```python
from build123d import *

# Parameters (mm, degrees)
SKETCH1_R                      = 6.35
BOSS_EXTRUDE1_DEPTH            = 54.102
SKETCH3_W                      = 6.35
SKETCH3_H                      = 14.605
CUT_EXTRUDE1_DEPTH             = 55.842241056
F_3_16_0_1875_DIAMETER_HOLE1_D = 4.7625
SKETCH7_RX                     = 6.35
SKETCH7_RY                     = 3.175
CUT_EXTRUDE2_DEPTH             = 56.532701566
CUT_EXTRUDE2_DEPTH_BACK        = 56.532701566
SKETCH9_W                      = 25.4
SKETCH9_H                      = 12.7


with BuildPart() as part:
    # Sketch1 → Boss-Extrude1 (new body)
    with BuildSketch(Plane(origin=(0, 0, 0), x_dir=(1, 0, 0), z_dir=(0, 1, 0))):
        with Locations(Location((0, 0, 0), (0, 0, 270))):
            Circle(SKETCH1_R)
    extrude(amount=BOSS_EXTRUDE1_DEPTH)

    # Sketch2 → Cut-Revolve1 (revolve, cut)
    with BuildSketch(Plane.XY, mode=Mode.PRIVATE) as cut_revolve1_sk:
        Polygon((26.057124612, 38.1), (6.35, 38.1), (2.54, 34.29), (2.54, 12.065), (6.35, 8.255), (26.057124612, 8.255), align=None)
    revolve(cut_revolve1_sk.sketch.rotate(Axis((0, 0, 0), (0, 1, 0)), 90), axis=Axis((0, 0, 0), (0, 1, 0)), mode=Mode.SUBTRACT)

    # Sketch3 → Cut-Extrude1 (cut, symmetric)
    with BuildSketch(Plane.XY):
        with Locations((7.62, 7.3025)):
            Rectangle(SKETCH3_W, SKETCH3_H)
    cut_extrude1 = extrude(amount=CUT_EXTRUDE1_DEPTH, both=True, mode=Mode.SUBTRACT)

    # Mirror1: Cut-Extrude1 across plane
    add(cut_extrude1.mirror(Plane(origin=(0, 0, 0), x_dir=(0, 0, 1), z_dir=(1, 0, 0))), mode=Mode.SUBTRACT)

    # 3/16 (0.1875) Diameter Hole1 (through all)
    with Locations(Plane.ZY.offset(4.445)):
        with Locations((0, 6.35)):
            Hole(F_3_16_0_1875_DIAMETER_HOLE1_D / 2)

    # Sketch7 → Cut-Revolve2 (revolve, cut)
    with BuildSketch(Plane.XY, mode=Mode.PRIVATE) as cut_revolve2_sk:
        with Locations(Location((7.9375, 46.1645), (0, 0, -90))):
            Ellipse(SKETCH7_RX, SKETCH7_RY)
    revolve(cut_revolve2_sk.sketch.rotate(Axis((0, 0, 0), (0, 1, 0)), 90), axis=Axis((0, 0, 0), (0, 1, 0)), mode=Mode.SUBTRACT)

    # Sketch8 → Cut-Revolve3 (revolve, cut)
    with BuildSketch(Plane(origin=(0, 0, 0), x_dir=(0, 0, -1), z_dir=(1, 0, 0))):
        with BuildLine():
            Line((4.7625, 54.102), (-4.7625, 54.102))
            ThreePointArc((-4.7625, 54.102), (0, 49.3395), (4.7625, 54.102))
        make_face()
    revolve(axis=Axis((0, 54.102, -4.7625), (0, 0, 1)), mode=Mode.SUBTRACT)

    # Sketch9 → Cut-Extrude2 (cut, two sides: drawn at the far end of the back side and taken through both)
    with BuildSketch(Plane(origin=(4.445, 0, 0), x_dir=(0, 0, -1), z_dir=(1, 0, 0)).offset(-CUT_EXTRUDE2_DEPTH_BACK)):
        with Locations((1.492425813, -3.81)):
            Rectangle(SKETCH9_W, SKETCH9_H)
    extrude(amount=CUT_EXTRUDE2_DEPTH + CUT_EXTRUDE2_DEPTH_BACK, mode=Mode.SUBTRACT)


solid = part.part
```
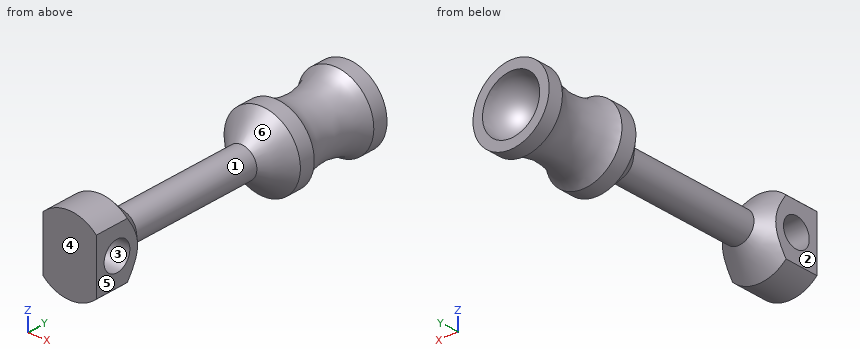
For this review, take the finished solid that the model builds, in its own axes (mm). Face numbers are marked on the shaded views. A direction names the side the tool comes from. Coordinates: 2 decimals unless noted, no trailing zeros. Write each loop counter-clockwise with the first axis right and the second up, starting at its lowest first coordinate (ties: lowest second). Pieces come first, ordered by that corner, then holes.
(1) The part is to be moulded in two halves that separate along Y. For the marked faces 4, 5 and 6, say which applies: +Y half, -Y half, draft (parallel to the pull), parting line (faces both ways), or undercut.
(2) Tool access review of the marked faces 1, 2 and 3: name each direction out of +Z, -Z, +X, -X, +Y, -Y from which nothing blocks a thin tool from reaching the whole face with its end or side.
(3) For pin 1 Ø1.5 at (x, y) = (1.5, 42) entering from +Z; pin 2 Ø3 at (x, y) = (0.5, 46.5) entering from -Z; pin 3 Ø2.5 at (y, z) = (8, -1.5) entering from -X (3 decimals); pin 4 Ø3 at (y, z) = (6.35, 0) entering from +X, all flat-tipped, find the tip position at first contact; note any pin that passes through.
(4) Add section B-B on x = 3.75. Count the separate pieces of the cut face and the enclosed holes in it, then the cut area to 3 significant figures.
(5) Add section C-C on y = 23. Give the boundary of the cut face in (x, z).
(6) Add section A-A on y = 6.35. Give the boundary of the cut face in (x, z) (3 decimals).
(7) Wall thickness on probe 1 along Y at (x, z) = (-3.75, 2) (3 decimals); probe 2 along Y at (x, z) = (-2.25, -1.5); probe 3 along Y at (x, z) = (0, 0): over which ranges is each line inside the solid? List them lowest first.
Answer sheet:
1. face 4: -Y half
1. face 5: draft
1. face 6: undercut
2. face 1: none
2. face 2: +Z, -Z, -X, -Y
2. face 3: +X, -X
3. pin 1: stops at z = 5.77
3. pin 2: stops at z = -4.89
3. pin 3: stops at x = -4.445
3. pin 4: passes through
4. separate pieces: 2
4. enclosed holes: 1
4. area: 192 mm2
5. outline: circle Ø5.08 at (0, 0)
6. outline: (-4.445, -4.535) arc R6.35 ccw to (4.445, -4.535) - (4.445, -2.381) - (-4.445, -2.381) - close; (-4.445, 2.381) - (4.445, 2.381) - (4.445, 4.535) arc R6.35 ccw to (-4.445, 4.535) - close
7. probe 1: y = 2.54 to 5.058, 7.642 to 10.355, 36 to 51.953
7. probe 2: y = 2.54 to 4.5, 8.2 to 11.9, 34.45 to 50.18
7. probe 3: y = 2.54 to 3.97, 8.73 to 49.34
